Here's the drawing with two shaded views (mm, measured from the low corner). I have some questions. A direction names the side the tool comes from. Give positions to 0.01 mm unless a question says otherwise; leave off trailing zeros. Loops run counter-clockwise (first coordinate to the right, second up) from the corner with the lowest first, then second, coordinate; pieces in that order, holes last. Notation, with made-up numbers: M 64,-25 L 76,-25 A23 cw 76,13 Z; hole C 70,45 d5. An arc over 180 degrees is marked long. Put each result on its own line as item: value. Start each with the question number.
1) For P1, Ø8, axis at x = 55, y = 5, coming from the +Z side (1 decimal), with a flat end and sliding along its axis, tell me the tip position at first contact or that it passes through.
2) For the marked faces 5 and 6, which set-ups out of +Z, -Z, +X, -X, +Y, -Y let a thin tool reach every point of the face, with its end or its side?
3) Please list where these lines run through material, in increasing order: line 1 along Y through (x, z) = (31.75, 1.8) (1 decimal); line 2 along X through (y, z) = (13, 28.5) (1 decimal); line 3 along Z through (x, y) = (8, 32.5) (1 decimal). Write a range as from..to.
4) Imagine slicing it at C-C (z = 36.5). Write out the boundary of the cut face in (x, y) (1 decimal).
5) Imagine slicing it at A-A (x = 31.75). Write out the boundary of the cut face in (y, z) (1 decimal).
6) If we mould it in two halves opening along X, with no side actions, what happens to the marked faces 1, 2, 3 and 4? For each: +X half, -X half, draft (parallel to the pull), parting line (faces both ways), or undercut.
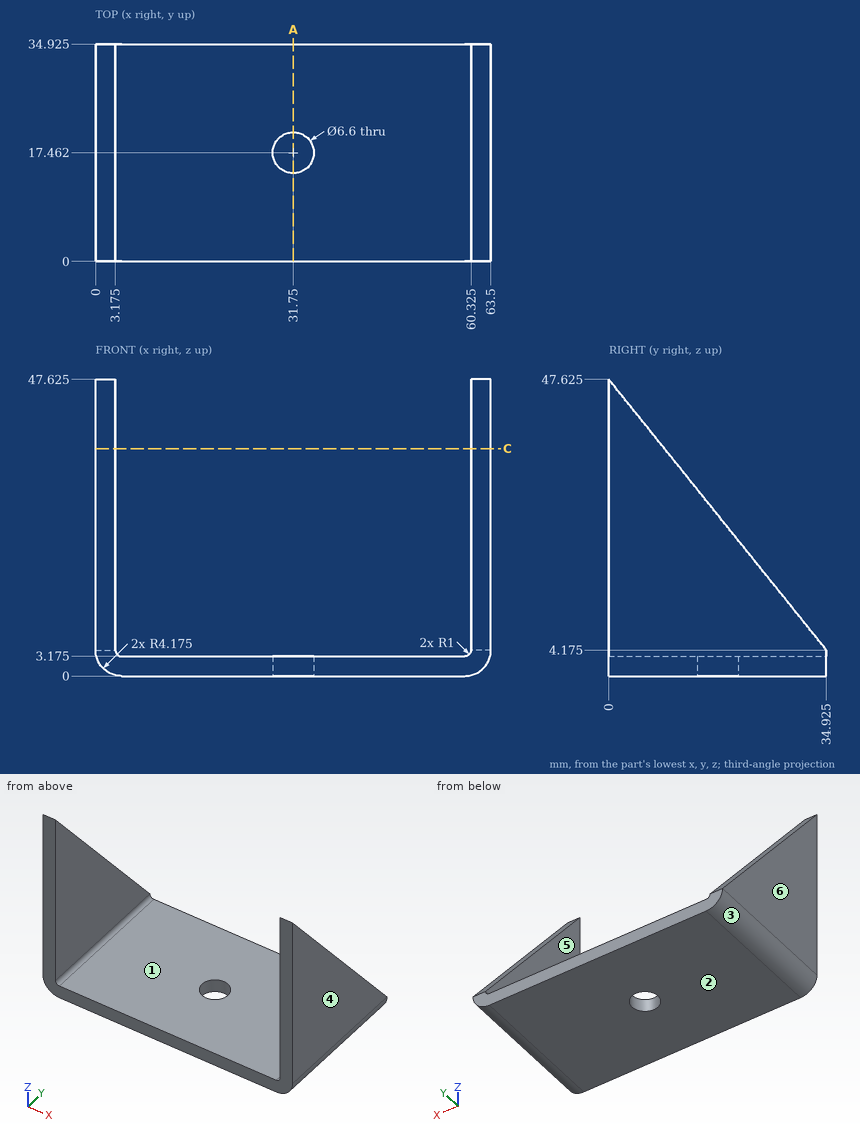
Recorded:
1. P1: z = 3.2
2. face 5: +Z, +Y, -Y
2. face 6: +Z, -Z, -X, +Y, -Y
3. line 1: 0..14.2, 20.8..34.9
3. line 2: 0..3.2, 60.3..63.5
3. line 3: 0..3.2
4. outline: M 0,0 L 3.2,0 L 3.2,8.9 L 0,8.9 Z; M 60.3,0 L 63.5,0 L 63.5,8.9 L 60.3,8.9 Z
5. outline: M 0,0 L 14.2,0 L 14.2,3.2 L 0,3.2 Z; M 20.8,0 L 34.9,0 L 34.9,3.2 L 20.8,3.2 Z
6. face 1: undercut
6. face 2: draft
6. face 3: -X half
6. face 4: +X half
